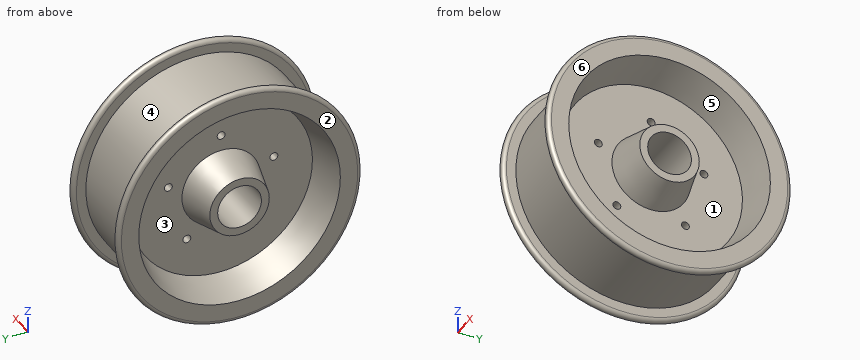
from build123d import *

# Parameters (mm, degrees)
F3_D = 6.35
F4_D = 6.35
F5_D = 6.35
F6_D = 6.35
F7_D = 6.35


with BuildPart() as f1:
    # F0 (on Front) → F1 (revolve)
    with BuildSketch(Plane.XZ):
        with BuildLine():
            Line((9.525, -11.215337), (9.525, 30.773766))
            Line((9.525, 30.773766), (38.1, 38.430415))
            Line((38.1, 38.430415), (38.1, 52.400415))
            ThreePointArc((38.1, 52.400415), (34.925, 55.575415), (31.75, 52.400415))
            Line((31.75, 52.400415), (31.75, 44.780415))
            Line((31.75, 44.780415), (-31.75, 44.780415))
            Line((-31.75, 44.780415), (-31.75, 52.400415))
            ThreePointArc((-31.75, 52.400415), (-34.925, 55.575415), (-38.1, 52.400415))
            Line((-38.1, 52.400415), (-38.1, 38.430415))
            Line((-38.1, 38.430415), (-9.525, 30.773766))
            Line((-9.525, 30.773766), (-9.525, -11.215337))
            Line((-9.525, -11.215337), (-38.1, -18.871985))
            Line((-38.1, -18.871985), (-38.1, -25.221985))
            Line((-38.1, -25.221985), (0, -25.221985))
            Line((0, -25.221985), (38.1, -25.221985))
            Line((38.1, -25.221985), (38.1, -18.871985))
            Line((38.1, -18.871985), (9.525, -11.215337))
        make_face()
    revolve(axis=Axis((44.160847, 0, -42.849585), (1, 0, 0)))

    # F3 (through all)
    with Locations(Plane.YZ.offset(9.525)):
        with Locations((-42.560316, -30.02687)):
            Hole(F3_D / 2)

    # F4 (through all)
    with Locations(Plane.YZ.offset(9.525)):
        with Locations((0, 1.600415)):
            Hole(F4_D / 2)

    # F5 (through all)
    with Locations(Plane.YZ.offset(9.525)):
        with Locations((-27.641779, -79.441398)):
            Hole(F5_D / 2)

    # F6 (through all)
    with Locations(Plane.YZ.offset(9.525)):
        with Locations((27.641779, -79.441398)):
            Hole(F6_D / 2)

    # F7 (through all)
    with Locations(Plane.YZ.offset(9.525)):
        with Locations((42.560316, -30.02687)):
            Hole(F7_D / 2)


solid = f1.part
Geometry check sheet. Reference: the model listing, model coordinates, mm. Face numbers are marked on the shaded views. A direction names the side the tool comes from. Give positions to 0.01 mm unless a question says otherwise; leave off trailing zeros. Write each loop counter-clockwise with the first axis right and the second up, starting at its lowest first coordinate (ties: lowest second). Pieces come first, ordered by that corner, then holes. Notation, with made-up numbers: M -5,32 L 36,32 A15 ccw 36,37 Z; hole C 38,-20.75 d5. An arc over 180 degrees is marked long. One line per question, with ' | ' between items.
1. Set-up check for the marked faces 1, 2 and 3: record each of +Z, -Z, +X, -X, +Y, -Y from which the full face is reachable in a straight line by a thin tool's end or side.
Ans:
face 1: +X | face 2: +Z, -Z, -X, +Y, -Y | face 3: -X
2. Scan lines: line 1 along Y through (x, z) = (-30, -67); line 2 along Z through (x, y) = (29.5, 5); line 3 along X through (y, z) = (-55.5, -116.5). Record each from-to range of solid material in increasing order. Write a range as from..to.
Ans:
line 1: -84.24..-75.33, -10.02..10.02, 75.33..84.24 | line 2: -130.34..-121.67, -68.65..-59.75, -25.95..-17.05, 35.97..44.64 | line 3: -38.1..-31.75, 31.75..38.1
3. Gauge pin test, flat ends, axial feed: pin 1 (8.5 mm diameter, centred on y = 27.64, z = -79.44, fed in from -X) (3 decimals); pin 2 (5 mm diameter, centred on y = -27.64, z = -79.44, fed in from +X); pin 3 (8 mm diameter, centred on x = 12, z = -25, fed in from -Y); pin 4 (5 mm diameter, centred on x = -10, y = -33.5, fed in from +Z). Record the tip position at first contact, or that the pin passes through.
Ans:
pin 1: x = -9.525 | pin 2: through | pin 3: y = -86.53 | pin 4: z = 39.11
4. Cross-section at B-B (y = 0). Count the separate pieces of the cut face and the enclosed holes in it, plus the area to 3 significant figures.
Ans:
separate pieces: 3 | enclosed holes: 0 | area: 5,130 mm2
5. Mould release check, pull along Z, two halves, no side actions. Record for the marked faces 4, 5 and 6: released by +Z, released by -Z, zero draft, split by the parting line, or undercut.
Ans:
face 4: split by the parting line | face 5: undercut | face 6: zero draft
6. Cross-section at A-A (x = -19). Enter the section's corners in (y, z), plus the area to 3 significant figures.
Ans:
outline: C 0,-42.85 d175.26; C 0,-42.85 d58.19; hole C 0,-42.85 d152.32; hole C 0,-42.85 d35.26 | area: 7,580 mm2
